Autodesk Inventor part; units mm, degrees
ref_plane "YZ Plane" through (0, 0, 0) normal (1, 0, 0) x (0, 1, 0)
ref_plane "XZ Plane" through (0, 0, 0) normal (0, 1, 0) x (-1, 0, 0)
ref_plane "XY Plane" through (0, 0, 0) normal (0, 0, 1) x (1, 0, 0)
sketch "草圖1" plane through (0, 0, 0) normal (0, 1, 0) x (-1, 0, 0)
  line L0 (-23.7, 13.54) -> (23.7, 13.54)
  line L1 (23.7, 13.54) -> (23.7, -13.54)
  line L2 (23.7, -13.54) -> (-23.7, -13.54)
  line L3 (-23.7, -13.54) -> (-23.7, 13.54)
  line L4 (-23.7, 13.54) -> (23.7, -13.54) construction
  line L5 (23.7, 13.54) -> (-23.7, -13.54) construction
  point P0 (0, 0)
  dimension "d0" = 47.4
  dimension "d1" = 27.08
extrude "擠出1" add sketch "草圖1" along normal blind 10.7
sketch "草圖2" plane through (23.7, 0, 13.54) normal (1, 0, 0) x (0, 0, -1)
  circle A0 centre (5.35, 5.35) radius 5.35
  line L0 (27.08, 10.7) -> (0, 10.7)
  line L1 (0, 0) -> (0, 10.7)
  point P0 (13.54, 0)
extrude "擠出2" add sketch "草圖2" along normal blind 100 contours A0
properties part number "telementry"
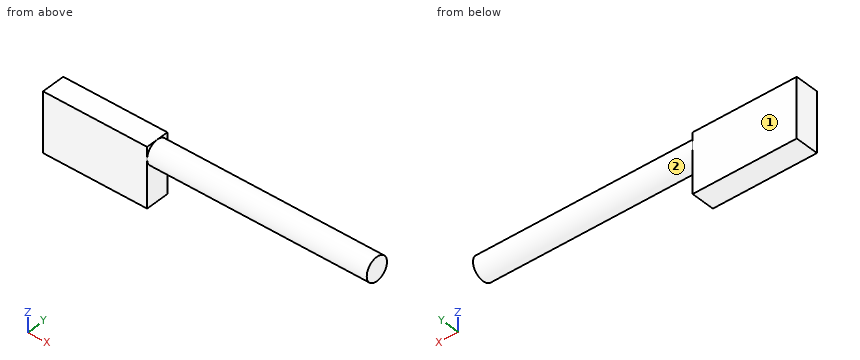
Geometry check sheet. Reference: the model listing, model coordinates, mm. Face numbers are marked on the shaded views. A direction names the side the tool comes from. Coordinates: 2 decimals unless noted, no trailing zeros. Loops run counter-clockwise (first coordinate to the right, second up) from the corner with the lowest first, then second, coordinate; pieces in that order, holes last.
Item 1: Access from +Z, -Z, +X, -X, +Y, -Y to the whole of each face (thin tool, end or side, straight path). Record for the marked faces 1 and 2.
Item 2: Thickness scan on line 1 (X direction, y = 8.75, z = 3); line 2 (Z direction, x = 63.5, y = 5.5); line 3 (Y direction, x = 104.5, z = 9.25). Record the ranges inside material, lowest first.
Item 3: Sectioned sample at C-C, the plane x = 40. Record the boundary of the cut face in (y, z), then the cut area to 3 significant figures.
Item 4: Sectioned sample at A-A, the plane y = 8.5. Record the boundary of the cut face in (x, z).
Item 5: Go/stop test with flat-tipped pins: pin 1 Ø12 at (x, z) = (97.5, -9) entering from +Y; pin 2 Ø3 at (x, y) = (71, 3.5) entering from +Z. Record where each tip stops, or that it passes through.
Item 6: Sectioned sample at B-B, the plane z = 6.5. Record the boundary of the cut face in (x, y).
Check result:
1. face 1: +Z, -Z, +X, -X, +Y
1. face 2: +X
2. line 1: x = -23.7 to 23.7
2. line 2: z = 2.84 to 13.54
2. line 3: y = 0.11 to 10.59
3. outline: circle Ø10.7 at (5.35, 8.19)
3. area: 89.9 mm2
4. outline: (-23.7, -13.54) - (23.7, -13.54) - (23.7, 3.87) - (123.7, 3.87) - (123.7, 12.51) - (23.7, 12.51) - (23.7, 13.54) - (-23.7, 13.54) - close
5. pin 1: passes through
5. pin 2: stops at z = 13.53
6. outline: (-23.7, 0) - (23.7, 0) - (23.7, 0.27) - (123.7, 0.27) - (123.7, 10.43) - (23.7, 10.43) - (23.7, 10.7) - (-23.7, 10.7) - close
